Part model, mm, in its own coordinate system. A direction names the side the tool comes from. Give positions to 0.01 mm unless a question says otherwise; leave off trailing zeros. Order: outer loops, then holes, each group sorted by start corner. A loop starts at its lowest first (then second) coordinate and runs counter-clockwise, first axis right, second up.
1. Slice it at A-A on z = 1.4. List the corners of the cut face in (x, y), and give its area (3 significant figures).
2. Probe line 1 (Y direction, x = -0.5, z = 1.55); line 2 (Y direction, x = -1, z = 0.9); line 3 (X direction, y = 1.75, z = 0.4). List the from-to ranges inside material, lowest first.
3. Drop flat-ended pins along their axis: pin 1 Ø2.5 at (x, y) = (-0.5, 8) entering from -Z; pin 2 Ø1.3 at (x, y) = (-0.5, -2) entering from -Z. Give the stop position or say it passes through.
4. Slice it at D-D on y = 8.25. List the corners of the cut face in (x, z).
5. Which spindle directions (+Z, -Z, +X, -X, +Y, -Y) get a long thin tool onto all of the face, cutting with end or side? Do faces 1 (the flat face through (4, -8, 1)), 2 (the flat face through (-3, 0, 1)). Say none if no direction does.
6. Mould opens along Y. For faces 3 (the flat face through (1, -10, 1)), 4 (the flat face through (0, 0, 2)), 5 (the cylindrical face through (0.06, 8.89, 1.01)) say: +Y half, -Y half, draft (parallel to the pull), parting line (faces both ways), or undercut.
7. Slice it at C-C on x = -0.5. List the corners of the cut face in (y, z).
8. Slice it at B-B on y = -2. List the corners of the cut face in (x, z).
from build123d import *

# Parameters (mm, degrees)
SKETCH_1_W          = 5
SKETCH_1_H          = 20
EXTRUDE_1_DEPTH     = 2
SKETCH_2_W          = 2.7
SKETCH_2_H          = 2
EXTRUDE_2_DEPTH     = 2
SKETCH_4_R          = 1.05
CUT_EXTRUDE_1_DEPTH = 2
SKETCH_5_R          = 1
CUT_EXTRUDE_2_DEPTH = 12
SKETCH_6_W          = 0.5
SKETCH_6_H          = 20
EXTRUDE_3_DEPTH     = 2


with BuildPart() as part:
    # 草图1 → 凸台-拉伸1 (new body)
    with BuildSketch(Plane.XY):
        Rectangle(SKETCH_1_W, SKETCH_1_H)
    extrude(amount=EXTRUDE_1_DEPTH)

    # 草图2 → 凸台-拉伸2 (add)
    with BuildSketch(Plane.XY.offset(2)):
        with Locations((3.85, -9)):
            Rectangle(SKETCH_2_W, SKETCH_2_H)
    extrude(amount=-EXTRUDE_2_DEPTH)

    # 草图4 → 切除-拉伸1 (cut)
    with BuildSketch(Plane.XY.offset(2)):
        with Locations((-0.5, -2)):
            Circle(SKETCH_4_R)
        with Locations((-0.5, 8)):
            Circle(SKETCH_4_R)
    extrude(amount=-CUT_EXTRUDE_1_DEPTH, mode=Mode.SUBTRACT)

    # 草图5 → 切除-拉伸2 (cut)
    with BuildSketch(Plane.XY.offset(2)):
        with Locations((2.5, -7)):
            Circle(SKETCH_5_R)
    extrude(amount=-CUT_EXTRUDE_2_DEPTH, mode=Mode.SUBTRACT)

    # 草图6 → 凸台-拉伸3 (add)
    with BuildSketch(Plane.XY.offset(2)):
        with Locations((-2.75, 0)):
            Rectangle(SKETCH_6_W, SKETCH_6_H)
    extrude(amount=-EXTRUDE_3_DEPTH)


solid = part.part
Data:
1. outline: (-3, -10) - (5.2, -10) - (5.2, -8) - (2.5, -8) arc R1 cw to (2.5, -6) - (2.5, 10) - (-3, 10) - close; hole circle Ø2.1 at (-0.5, -2); hole circle Ø2.1 at (-0.5, 8)
1. area: 107 mm2
2. line 1: y = -10 to -3.05, -0.95 to 6.95, 9.05 to 10
2. line 2: y = -10 to -2.92, -1.08 to 7.08, 8.92 to 10
2. line 3: x = -3 to 2.5
3. pin 1: stops at z = 0
3. pin 2: passes through
4. outline: (-3, 0) - (-1.52, 0) - (-1.52, 2) - (-3, 2) - close; (0.52, 0) - (2.5, 0) - (2.5, 2) - (0.52, 2) - close
5. face 1: +Z, -Z, +X, +Y
5. face 2: +Z, -Z, -X, +Y, -Y
6. face 3: -Y half
6. face 4: draft
6. face 5: undercut
7. outline: (-10, 0) - (-3.05, 0) - (-3.05, 2) - (-10, 2) - close; (-0.95, 0) - (6.95, 0) - (6.95, 2) - (-0.95, 2) - close; (9.05, 0) - (10, 0) - (10, 2) - (9.05, 2) - close
8. outline: (-3, 0) - (-1.55, 0) - (-1.55, 2) - (-3, 2) - close; (0.55, 0) - (2.5, 0) - (2.5, 2) - (0.55, 2) - close
